Design review of the part built by this model. Coordinates are the model's own, in mm. Face numbers are marked on the shaded views. Coordinates: 2 decimals unless noted, no trailing zeros. Write each loop counter-clockwise with the first axis right and the second up, starting at its lowest first coordinate (ties: lowest second). Pieces come first, ordered by that corner, then holes.
Q1. Insertion check: pin 1 (2 mm diameter, centred on y = 44.5, z = 64, fed in from +X); pin 2 (1.6 mm diameter, centred on y = 44.5, z = 65, fed in from -X); pin 3 (2 mm diameter, centred on x = -142.5, y = 57.5, fed in from -Z); pin 4 (8 mm diameter, centred on x = -167, z = 24.5, fed in from -Y). Each pin has a flat end and moves straight along its axis. Give the tip position at first contact, or say it passes through.
Q2. Take a section at A-A (x = -70). Give the boundary of the cut face in (y, z), and give its area (3 significant figures).
Q3. Take a section at C-C (x = -156.5). Give the boundary of the cut face in (y, z), and give its area (3 significant figures).
Q4. For probe 1 along Y at (x, z) = (-70, 2); probe 2 along Z at (x, y) = (-125, 46); probe 3 along X at (y, z) = (49.8, 64.75), list the stretches that pass through material, from the lowest coordinate up.
Q5. Take a section at B-B (y = 49.8). Give the boundary of the cut face in (x, z), and give its area (3 significant figures).
Q6. Take a section at D-D (z = 30.5). Give the boundary of the cut face in (x, y), and give its area (3 significant figures).
Q7. Mouldability with a two-part tool opening along Z and no side actions: class the marked faces 1, 2 and 3 as pulls with the +Z half, pulls with the -Z half, needs draft (parallel to the pull), parting line crosses it, or undercut.
```python
from build123d import *

# Parameters (mm, degrees)
SKETCH1_W           = 132.917449813
SKETCH1_H           = 12
SKETCH1_R           = 2.55
BOSS_EXTRUDE1_DEPTH = 4
SKETCH2_W           = 197.917449813
SKETCH2_H           = 67
BOSS_EXTRUDE2_DEPTH = 4
BOSS_EXTRUDE3_START = 4
SKETCH3_W           = 132.917449813
SKETCH3_H           = 12
SKETCH3_R           = 2.55
BOSS_EXTRUDE3_DEPTH = 4
FILLET1_R           = 10
FILLET2_R           = 2.5


with BuildPart() as part:
    # Sketch1 → Boss-Extrude1 (new body)
    with BuildSketch(Plane.XY):
        with Locations((-116.458724907, 49.8)):
            Rectangle(SKETCH1_W, SKETCH1_H)
        with Locations((-162.917449813, 49.8)):
            Circle(SKETCH1_R, mode=Mode.SUBTRACT)
        with Locations((-70, 49.8)):
            Circle(SKETCH1_R, mode=Mode.SUBTRACT)
    extrude(amount=BOSS_EXTRUDE1_DEPTH)

    # Sketch2 → Boss-Extrude2 (add)
    with BuildSketch(Plane(origin=(0, 55.8, 0), x_dir=(1, 0, 0), z_dir=(0, 1, 0))):
        with Locations((-108.958724907, -33.5)):
            Rectangle(SKETCH2_W, SKETCH2_H)
    extrude(amount=BOSS_EXTRUDE2_DEPTH)

    # Sketch3 → Boss-Extrude3 (add)
    with BuildSketch(Plane(origin=(0, 0, 67), x_dir=(-1, 0, 0), z_dir=(0, 0, -1)).offset(BOSS_EXTRUDE3_START)):
        with Locations((116.458724907, 49.8)):
            Rectangle(SKETCH3_W, SKETCH3_H)
        with Locations(Location((162.917449813, 49.8, 0), (0, 0, 180))):
            Circle(SKETCH3_R, mode=Mode.SUBTRACT)
        with Locations(Location((70, 49.8, 0), (0, 0, 180))):
            Circle(SKETCH3_R, mode=Mode.SUBTRACT)
    extrude(amount=-BOSS_EXTRUDE3_DEPTH)

    # Fillet1
    fillet1_edges = [part.edges().sort_by_distance(p)[0] for p in [
        (-182.917449813, 55.8, 65),
        (-50, 55.8, 65),
        (-182.917449813, 55.8, 2),
        (-50, 55.8, 2),
    ]]
    fillet(fillet1_edges, radius=FILLET1_R)

    # Fillet2
    fillet2_edges = [part.edges().sort_by_distance(p)[0] for p in [
        (-116.458724906, 55.8, 4),
        (-116.458724906, 55.8, 63),
    ]]
    fillet(fillet2_edges, radius=FILLET2_R)


solid = part.part
```
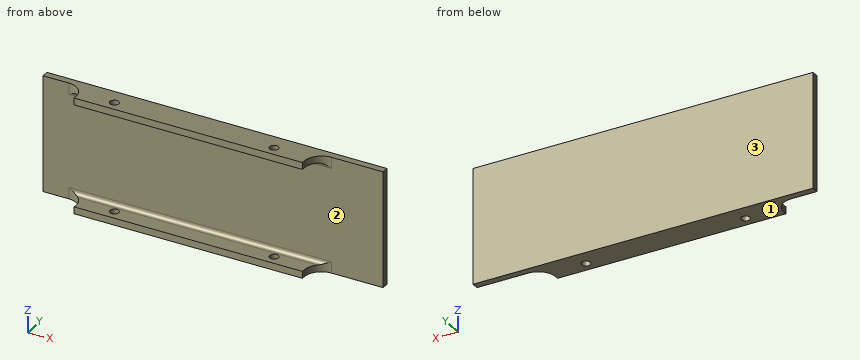
Response:
1. pin 1: stops at x = -50
1. pin 2: stops at x = -182.92
1. pin 3: stops at z = 0
1. pin 4: stops at y = 55.8
2. outline: (43.8, 0) - (47.25, 0) - (47.25, 4) - (43.8, 4) - close; (43.8, 63) - (47.25, 63) - (47.25, 67) - (43.8, 67) - close; (52.35, 0) - (59.8, 0) - (59.8, 67) - (52.35, 67) - (52.35, 63) - (53.3, 63) arc R2.5 cw to (55.8, 60.5) - (55.8, 6.5) arc R2.5 cw to (53.3, 4) - (52.35, 4) - close
2. area: 326 mm2
3. outline: (43.8, 0) - (59.8, 0) - (59.8, 67) - (43.8, 67) - (43.8, 63) - (53.3, 63) arc R2.5 cw to (55.8, 60.5) - (55.8, 6.5) arc R2.5 cw to (53.3, 4) - (43.8, 4) - close
3. area: 367 mm2
4. probe 1: y = 43.8 to 47.25, 52.35 to 59.8
4. probe 2: z = 0 to 4, 63 to 67
4. probe 3: x = -183.75 to -165.47, -160.37 to -72.55, -67.45 to -49.17
5. outline: (-183.75, 0) - (-165.47, 0) - (-165.47, 4) - (-183.75, 4) - close; (-183.75, 63) - (-165.47, 63) - (-165.47, 67) - (-183.75, 67) - close; (-160.37, 0) - (-72.55, 0) - (-72.55, 4) - (-160.37, 4) - close; (-160.37, 63) - (-72.55, 63) - (-72.55, 67) - (-160.37, 67) - close; (-67.45, 0) - (-49.17, 0) - (-49.17, 4) - (-67.45, 4) - close; (-67.45, 63) - (-49.17, 63) - (-49.17, 67) - (-67.45, 67) - close
5. area: 995 mm2
6. outline: (-207.92, 55.8) - (-10, 55.8) - (-10, 59.8) - (-207.92, 59.8) - close
6. area: 792 mm2
7. face 1: pulls with the -Z half
7. face 2: undercut
7. face 3: needs draft
